Part model, mm, in its own coordinate system. A direction names the side the tool comes from. Round coordinates to 2 decimals unless told otherwise and drop trailing zeros. Write each loop counter-clockwise with the first axis right and the second up, starting at its lowest first coordinate (ties: lowest second). Pieces come first, ordered by that corner, then holes.
1) Flat gauge pins, fed straight in: pin 1 (2 mm diameter, centred on y = 6.5, z = 2, fed in from +X); pin 2 (3 mm diameter, centred on y = 2, z = -0.5, fed in from -X); pin 3 (5 mm diameter, centred on y = 12, z = 2, fed in from -X). Where does each tip first touch, or does it go through?
2) Pull direction Z, two halves, no side cores. Call faces 1 (the flat face through (-5, 14, 9.5)), 2 (the flat face through (6.65, 13.59, 10.01)), 3 (the flat face through (0, 7, 0)): +Z half, -Z half, draft (parallel to the pull), parting line (faces both ways), or undercut.
3) Saw through at C-C on y = 5.75. Write the cut outline in (x, z), and give its area (3 significant figures).
4) Saw through at B-B on y = 8. Write the cut outline in (x, z).
5) Saw through at A-A on x = 0. Write the cut outline in (y, z).
6) Saw through at D-D on z = 6. Write the cut outline in (x, y).
7) Which spindle directions (+Z, -Z, +X, -X, +Y, -Y) get a long thin tool onto all of the face, cutting with end or side? Do faces 4 (the flat face through (-9.6, 3.7, -7.1)), 5 (the flat face through (-8, 4, 7.5)), 6 (the flat face through (9, 3, 7.5)), 7 (the flat face through (5, 13, 10)). Say none if no direction does.
8) Drill centre lines: L1, parallel to X at y = 5.5, z = 0; L2, parallel to X at y = 19, z = 8.75; L3, parallel to X at y = 3, z = -2.5. Where is each one in solid material? Low to high.
```python
from build123d import *

# Parameters (mm, degrees)
SKETCH1_W           = 20
SKETCH1_H           = 15
BOSS_EXTRUDE1_DEPTH = 20
SKETCH2_R           = 4.5
CUT_EXTRUDE1_DEPTH  = 7
BOSS_EXTRUDE2_DEPTH = 3
CUT_EXTRUDE4_DEPTH  = 1
FILLET1_R           = 2
WRAP1_SECTION_W     = 0.5
WRAP1_SECTION_H     = 15
WRAP1_ANGLE         = 42.971834635


# Read off the part's stored shape, not the designer's step: Dome1
with BuildPart() as part:
    # Sketch1 → Boss-Extrude1 (new body)
    with BuildSketch(Plane(origin=(0, 0, 0), x_dir=(1, 0, 0), z_dir=(0, 1, 0))):
        Rectangle(SKETCH1_W, SKETCH1_H)
    extrude(amount=BOSS_EXTRUDE1_DEPTH)

    # Sketch2 → Cut-Extrude1 (cut)
    with BuildSketch(Plane.XZ):
        with Locations(Location((0, 0, 0), (0, 0, 270))):
            Circle(SKETCH2_R)
    extrude(amount=-CUT_EXTRUDE1_DEPTH, mode=Mode.SUBTRACT)

    # Sketch3 → Boss-Extrude2 (add)
    with BuildSketch(Plane.XY.offset(7.5)):
        Polygon((-10, 20), (-10, 10), (-5.5, 0), (5.5, 0), (10, 10), (10, 20), align=None)
    extrude(amount=BOSS_EXTRUDE2_DEPTH)

    # Sketch5 → Cut-Extrude4 (cut)
    with BuildSketch(Plane.XY.offset(10.5)):
        Polygon((-7, 14.2), (-4, 14.2), (-3.307179677, 13), (-6.307179677, 13), align=None)
    cut_extrude4 = extrude(amount=-CUT_EXTRUDE4_DEPTH, mode=Mode.SUBTRACT)

    # Mirror2: Cut-Extrude4 across plane
    add(cut_extrude4.mirror(Plane(origin=(0, 0, 0), x_dir=(0, 0, 1), z_dir=(1, 0, 0))), mode=Mode.SUBTRACT)

    # Dome1 outline → Dome1 (revolve)
    with BuildSketch(Plane(origin=(0, 14, 0), x_dir=(0, 1, 0), z_dir=(0, 0, -1))):
        with BuildLine():
            Line((0, -9.9999999), (0, -13))
            add(Edge.make_bspline(
                [(0, -13), (4.5, -13), (4.5, -10)],
                knots=[4.71238898, 4.71238898, 4.71238898, 6.283185307, 6.283185307, 6.283185307], degree=2, weights=[1, 0.707106781, 1]))
            Line((4.5, -10), (0, -9.9999999))
        make_face()
    dome1 = revolve(axis=Axis((0, 14, 0), (1, 0, 0)))

    # Mirror7: Dome1 across plane
    add(dome1.mirror(Plane(origin=(0, 0, 0), x_dir=(0, 0, 1), z_dir=(1, 0, 0))))

    # Fillet1
    fillet1_edges = [part.edges().sort_by_distance(p)[0] for p in [
        (-10, 10, -7.5),
        (10, 10, -7.5),
    ]]
    fillet(fillet1_edges, radius=FILLET1_R)

    # Wrap1 section (on wrap section) → Wrap1 (revolve)
    with BuildSketch(Plane(origin=(8, 0, -5.5), x_dir=(0.9169620384790573, 0, -0.39897446032087286), z_dir=(0.39897446032087286, 0, 0.9169620384790573))):
        with Locations((2.25, 11.2)):
            Rectangle(WRAP1_SECTION_W, WRAP1_SECTION_H)
    wrap1 = revolve(axis=Axis((8, 0, -5.5), (0, 1, 0)), revolution_arc=WRAP1_ANGLE)

    # Mirror9: Wrap1 across plane
    add(wrap1.mirror(Plane(origin=(0, 0, 0), x_dir=(0, 0, 1), z_dir=(1, 0, 0))))


solid = part.part
```
Completed:
1. pin 1: stops at x = 10
1. pin 2: stops at x = -10
1. pin 3: stops at x = -12.99
2. face 1: +Z half
2. face 2: draft
2. face 3: undercut
3. outline: (-10.29, -6.5) arc R2.5 ccw to (-9, -7.79) - (-8.8, -7.33) arc R2 ccw to (-8, -7.5) - (8, -7.5) arc R2 ccw to (8.8, -7.33) - (9, -7.79) arc R2.5 ccw to (10.29, -6.5) - (9.83, -6.3) arc R2 ccw to (10, -5.5) - (10, 7.5) - (8.09, 7.5) - (8.09, 10.5) - (-8.09, 10.5) - (-8.09, 7.5) - (-10, 7.5) - (-10, -5.5) arc R2 ccw to (-9.83, -6.3) - close; hole circle Ø9 at (0, 0)
3. area: 285 mm2
4. outline: (-10.29, -6.5) arc R2.5 ccw to (-9, -7.79) - (-8.8, -7.33) arc R2 ccw to (-8, -7.5) - (8, -7.5) arc R2 ccw to (8.8, -7.33) - (9, -7.79) arc R2.5 ccw to (10.29, -6.5) - (9.83, -6.3) arc R2 ccw to (10, -5.5) - (10, 7.5) - (9.1, 7.5) - (9.1, 10.5) - (-9.1, 10.5) - (-9.1, 7.5) - (-10, 7.5) - (-10, -5.5) arc R2 ccw to (-9.83, -6.3) - close
5. outline: (0, -7.5) - (20, -7.5) - (20, 10.5) - (0, 10.5) - (0, 4.5) - (7, 4.5) - (7, -4.5) - (0, -4.5) - close
6. outline: (-10, 0) - (10, 0) - (10, 20) - (-10, 20) - close
7. face 4: -Z, -X, -Y
7. face 5: +Z, -X, -Y
7. face 6: +Z, +X, -Y
7. face 7: +Z
8. L1: x = -10 to -4.5, 4.5 to 10
8. L2: x = -10 to 10
8. L3: x = -10 to -3.74, 3.74 to 10
